```python
from build123d import *

# Parameters (mm, degrees)
F0_R      = 17
F1_DEPTH  = 10
F2_R      = 8.5
F3_DEPTH  = 8
F4_R      = 6.5
F5_DEPTH  = 2.001
F7_DEPTH  = 12.5
F10_R     = 3.85
F11_DEPTH = 1.5
F12_R     = 3.85
F13_DEPTH = 1.5
F15_R     = 2.55
F16_DEPTH = 34.5010001


# Not quite as in the source:
# - a fillet or chamfer that OpenCascade refuses, or shapes differently, is made with other operations: its cross-section is extruded or revolved along the edge and cut away or added


with BuildPart() as f1:
    # F0 (on Top) → F1 (new body)
    with BuildSketch(Plane.XY):
        Circle(F0_R)
    extrude(amount=F1_DEPTH)

    # F2 (on face) → F3 (cut)
    with BuildSketch(Plane.XY.offset(10)):
        Circle(F2_R)
    extrude(amount=-F3_DEPTH, mode=Mode.SUBTRACT)

    # F4 (on face) → F5 (cut, through all)
    with BuildSketch(Plane.XY.offset(2)):
        Circle(F4_R)
    extrude(amount=-F5_DEPTH, mode=Mode.SUBTRACT)

    # F6 (on Front) → F7 (cut, symmetric)
    with BuildSketch(Plane.XZ):
        Polygon((4.6188021535, 6), (2.3094010768, 10), (-2.3094010768, 10), (-4.6188021535, 6), (-2.3094010768, 2), (2.3094010768, 2), align=None)
    extrude(amount=F7_DEPTH, both=True, mode=Mode.SUBTRACT)

    # F10 (on offset) → F11 (cut)
    with BuildSketch(Plane.XZ.offset(17.5)):
        with Locations((0, 6)):
            Circle(F10_R)
    extrude(amount=-F11_DEPTH, mode=Mode.SUBTRACT)

    # F12 (on offset) → F13 (cut)
    with BuildSketch(Plane.XZ.offset(-17.5)):
        with Locations((0, 6)):
            Circle(F12_R)
    extrude(amount=F13_DEPTH, mode=Mode.SUBTRACT)

    # F14: fillet of radius 5 on 1 edges, made by hand

    # F14_s1 → F14_t2 (revolve, cut)
    with BuildSketch(Plane.XZ):
        with BuildLine():
            ThreePointArc((17, 5), (15.5355339059, 1.4644660941), (12, 0))
            Line((12, 0), (17, 0))
            Line((17, 0), (17, 5))
        make_face()
    revolve(axis=Axis((0, 0, 0), (0, 0, 1)), mode=Mode.SUBTRACT)

    # F15 (on offset) → F16 (cut, through all)
    with BuildSketch(Plane.XZ.offset(17.5)):
        with Locations((0, 6)):
            Circle(F15_R)
    extrude(amount=-F16_DEPTH, mode=Mode.SUBTRACT)


solid = f1.part
```
Work out the finished part from the listing and answer in its coordinate system (mm). A direction names the side the tool comes from. Give positions to 0.01 mm unless a question says otherwise; leave off trailing zeros. Order: outer loops, then holes, each group sorted by start corner. A loop starts at its lowest first (then second) coordinate and runs counter-clockwise, first axis right, second up.
1. The mould has two halves that part along Z. Classify faces 1 (the flat face through (5, -5, 0)), 2 (the flat face through (-8, -4, 10)), 3 (the cylindrical face through (2.43, -14.27, 6.77)): released by +Z, released by -Z, zero draft, split by the parting line, or undercut.
Result sheet:
face 1: released by -Z
face 2: released by +Z
face 3: undercut
2. Section B-B, the plane x = 0 is taken. Determine the outline of the cut face in (y, z), and give its area (3 significant figures).
Result sheet:
outline: (-17, 9.85) - (-16, 9.85) - (-16, 8.55) - (-12.5, 8.55) - (-12.5, 10) - (-17, 10) - close; (-16.11, 2.15) arc R5 ccw to (-12, 0) - (-6.5, 0) - (-6.5, 2) - (-12.5, 2) - (-12.5, 3.45) - (-16, 3.45) - (-16, 2.15) - close; (6.5, 0) - (12, 0) arc R5 ccw to (16.11, 2.15) - (16, 2.15) - (16, 3.45) - (12.5, 3.45) - (12.5, 2) - (6.5, 2) - close; (12.5, 8.55) - (16, 8.55) - (16, 9.85) - (17, 9.85) - (17, 10) - (12.5, 10) - close
area: 53.8 mm2
3. Section A-A, the plane y = 0 is taken. Determine the outline of the cut face in (x, z), and give its area (3 significant figures).
Result sheet:
outline: (-17, 5) arc R5 ccw to (-12, 0) - (-6.5, 0) - (-6.5, 2) - (-8.5, 2) - (-8.5, 10) - (-17, 10) - close; (6.5, 0) - (12, 0) arc R5 ccw to (17, 5) - (17, 10) - (8.5, 10) - (8.5, 2) - (6.5, 2) - close
area: 167 mm2
4. Each of these flat-tipped pins is pushed along its axis until it touches: P1, Ø6, axis at x = 4, z = 2, coming from the +Y side; P2, Ø12, axis at x = -6.5, y = 2.5, coming from the +Z side; P3, Ø1, axis at x = 11.5, z = 7.5, coming from the -Y side; P4, Ø6, axis at y = 6.5, z = 5.5, coming from the -X side. Where does it stop, or does it pass through?
Result sheet:
P1: stops at y = 16.6
P2: stops at z = 10
P3: stops at y = -12.96
P4: stops at x = -16.64
5. For faces 4 (the flat face through (1, -16, 3)), 5 (the flat face through (1, 7, 2)), 6 (the flat face through (-3.48, -9.86, 4.03)), determine the directions among +Z, -Z, +X, -X, +Y, -Y from which every point of the face is accessible in a straight line to the end or side of a thin tool.
Result sheet:
face 4: -Y
face 5: +Z
face 6: none
6. Straight lines are drawn through the part: L1, parallel to Y at x = 0, z = 3; L2, parallel to Y at x = -2.5, z = 1.75; L3, parallel to X at y = -4.5, z = 6.5. For each, find the intervals that lie inside material, in ascending order.
Result sheet:
L1: y = -16 to -12.5, 12.5 to 16
L2: y = -15.6 to -6, 6 to 15.6
L3: x = -16.39 to -7.21, 7.21 to 16.39
